from build123d import *

# Parameters (mm, degrees)
BOSS_EXTRUDE1_DEPTH = 25
SKETCH2_R           = 3
BOSS_EXTRUDE2_DEPTH = 1
SKETCH3_R           = 1
BOSS_EXTRUDE3_DEPTH = 8
BOSS_EXTRUDE4_DEPTH = 2
BOSS_EXTRUDE5_START = 0.5
SKETCH5_R           = 1
BOSS_EXTRUDE5_DEPTH = 0.5
FILLET1_R           = 1
FILLET2_R           = 1


with BuildPart() as part:
    # Sketch1 → Boss-Extrude1 (new body)
    with BuildSketch(Plane.XY):
        with BuildLine():
            Line((-7.5, -6.614378278), (-7.5, 6.614378278))
            ThreePointArc((-7.5, 6.614378278), (0, 10), (7.5, 6.614378278))
            Line((7.5, 6.614378278), (7.5, -6.614378278))
            ThreePointArc((7.5, -6.614378278), (0, -10), (-7.5, -6.614378278))
        make_face()
    extrude(amount=BOSS_EXTRUDE1_DEPTH)

    # Sketch2 → Boss-Extrude2 (add)
    with BuildSketch(Plane.XY.offset(25)):
        Circle(SKETCH2_R)
    extrude(amount=BOSS_EXTRUDE2_DEPTH)

    # Sketch3 → Boss-Extrude3 (add)
    with BuildSketch(Plane.XY.offset(26)):
        Circle(SKETCH3_R)
    extrude(amount=BOSS_EXTRUDE3_DEPTH)

    # Sketch4 → Boss-Extrude4 (add)
    with BuildSketch(Plane(origin=(0, 0, 0), x_dir=(-1, 0, 0), z_dir=(0, 0, -1))):
        with BuildLine():
            Line((4, 3), (4, -3))
            ThreePointArc((4, -3), (-5, 0), (4, 3))
        make_face()
    extrude(amount=BOSS_EXTRUDE4_DEPTH)

    # Sketch5 → Boss-Extrude5 (add)
    with BuildSketch(Plane(origin=(0, 0, -2), x_dir=(-1, 0, 0), z_dir=(0, 0, -1)).offset(BOSS_EXTRUDE5_START)):
        with Locations(Location((0, 0, 0), (0, 0, 180))):
            Circle(SKETCH5_R)
    extrude(amount=-BOSS_EXTRUDE5_DEPTH)

    # Fillet1
    fillet1_edges = [part.edges().sort_by_distance(p)[0] for p in [
        (0, -10, 25),
        (7.5, 0, 25),
        (0, 10, 25),
        (-7.5, 0, 25),
    ]]
    fillet(fillet1_edges, radius=FILLET1_R)

    # Fillet2
    fillet2_edges = [part.edges().sort_by_distance(p)[0] for p in [
        (7.5, 0, 0),
        (0, -10, 0),
        (-7.5, 0, 0),
        (0, 10, 0),
    ]]
    fillet(fillet2_edges, radius=FILLET2_R)


solid = part.part
Can you work these out from the model? Positions are in its coordinate system, mm. A direction names the side the tool comes from. Give positions to 0.01 mm unless a question says otherwise; leave off trailing zeros. Loops run counter-clockwise (first coordinate to the right, second up) from the corner with the lowest first, then second, coordinate; pieces in that order, holes last. Notation, with made-up numbers: (74.5, 50.25) -> (97.5, 50.25) arc R20 cw to (97.5, 87.25) -> close; hole circle Ø5 at (0, 11). An arc over 180 degrees is marked (long way). Use one line per item in the form item = value.
1) If we section it at A-A (x = 0): Please give me the cut outline in (y, z), plus the area to 3 significant figures.
Answers:
outline = (-10, 1) arc R1 ccw to (-9, 0) -> (-5, 0) -> (-5, -2) -> (-1, -2) -> (-1, -2.5) -> (1, -2.5) -> (1, -2) -> (5, -2) -> (5, 0) -> (9, 0) arc R1 ccw to (10, 1) -> (10, 24) arc R1 ccw to (9, 25) -> (3, 25) -> (3, 26) -> (1, 26) -> (1, 34) -> (-1, 34) -> (-1, 26) -> (-3, 26) -> (-3, 25) -> (-9, 25) arc R1 ccw to (-10, 24) -> close
area = 542 mm²
2) For faces 1 (the face through (0, -10, 12)), 2 (the face through (-4.2, 0.1, 0)), 3 (the face through (0, -1, 30)), 4 (the face through (0, 0, 34)), 5 (the face through (-4, 0, -1)), which set-ups out of +Z, -Z, +X, -X, +Y, -Y let a thin tool reach every point of the face, with its end or its side?
Answers:
face_1 = +Z, -Z, -Y
face_2 = -Z
face_3 = +Z
face_4 = +Z, +X, -X, +Y, -Y
face_5 = -Z, -X, +Y, -Y
3) If we section it at C-C (z = 16.5): Please give me the cut outline in (x, y).
Answers:
outline = (-7.5, -6.61) arc R10 ccw to (7.5, -6.61) -> (7.5, 6.61) arc R10 ccw to (-7.5, 6.61) -> close
4) I need wall thicknesses on line 1 along Z through (x, y) = (-6.25, -5.25); line 2 along Z through (x, y) = (2.5, 1.25); line 3 along X through (y, z) = (7.5, 23). Which ranges of each line are inside material? Lowest first, please.
Answers:
line_1 = 0 to 25
line_2 = -2 to 26
line_3 = -6.61 to 6.61
5) If we section it at B-B (y = 0): Please give me the cut outline in (x, z).
Answers:
outline = (-7.5, 1) arc R1 ccw to (-6.5, 0) -> (-4, 0) -> (-4, -2) -> (-1, -2) -> (-1, -2.5) -> (1, -2.5) -> (1, -2) -> (5, -2) -> (5, 0) -> (6.5, 0) arc R1 ccw to (7.5, 1) -> (7.5, 24) arc R1 ccw to (6.5, 25) -> (3, 25) -> (3, 26) -> (1, 26) -> (1, 34) -> (-1, 34) -> (-1, 26) -> (-3, 26) -> (-3, 25) -> (-6.5, 25) arc R1 ccw to (-7.5, 24) -> close
6) Will these pins go through, and if not, where does the flat tip stop? pin 1 (3 mm diameter, centred on x = 2.5, y = 7, fed in from -Z); pin 2 (5 mm diameter, centred on x = 3.5, y = 2, fed in from -Z); pin 3 (0.6 mm diameter, centred on y = -0.5, z = -1, fed in from -X).
Answers:
pin_1 = 0
pin_2 = -2
pin_3 = -4
7) If we section it at D-D (y = 4.25): Please give me the cut outline in (x, z), plus the area to 3 significant figures.
Answers:
outline = (-7.5, 1) arc R1 ccw to (-6.5, 0) -> (-2.63, 0) -> (-2.63, -2) -> (2.63, -2) -> (2.63, 0) -> (6.5, 0) arc R1 ccw to (7.5, 1) -> (7.5, 24) arc R1 ccw to (6.5, 25) -> (-6.5, 25) arc R1 ccw to (-7.5, 24) -> close
area = 385 mm²
